```python
from build123d import *

# Parameters (mm, degrees)
F0_R     = 1.75
F1_DEPTH = 12
F2_R     = 1.75
F3_DEPTH = 15


with BuildPart() as f1:
    # F0 (on Top) → F1 (new body)
    with BuildSketch(Plane.XY):
        Polygon((160, 0), (0, 0), (0, -25), (42, -25), (42, -120), (110, -120), (110, -50), (160, -50), align=None)
        with Locations((49, -113)):
            Circle(F0_R, mode=Mode.SUBTRACT)
        with Locations((103, -113)):
            Circle(F0_R, mode=Mode.SUBTRACT)
        with Locations((49, -59)):
            Circle(F0_R, mode=Mode.SUBTRACT)
        with Locations((9, -12.5)):
            Circle(F0_R, mode=Mode.SUBTRACT)
        with Locations((103, -59)):
            Circle(F0_R, mode=Mode.SUBTRACT)
        with Locations((111, -12.5)):
            Circle(F0_R, mode=Mode.SUBTRACT)
        with Locations((141, -8)):
            Circle(F0_R, mode=Mode.SUBTRACT)
    extrude(amount=F1_DEPTH)

    # F2 (on face) → F3 (cut)
    with BuildSketch(Plane(origin=(0, 0, 0), x_dir=(-1, 0, 0), z_dir=(0, 1, 0))):
        with Locations((-156, 6)):
            Circle(F2_R)
        with Locations((-84, 6)):
            Circle(F2_R)
        with Locations((-13, 6)):
            Circle(F2_R)
    extrude(amount=-F3_DEPTH, mode=Mode.SUBTRACT)


solid = f1.part
```
Could you check a few things on this model? Use its own coordinates, in mm. A direction names the side the tool comes from. Give positions to 0.01 mm unless a question says otherwise; leave off trailing zeros. Order: outer loops, then holes, each group sorted by start corner. A loop starts at its lowest first (then second) coordinate and runs counter-clockwise, first axis right, second up.
Q1. For faces 1 (the flat face through (42, -72, 6)), 2 (the flat face through (135, -50, 6)), 3 (the cylindrical face through (82.331, -7.395, 6.526)), which set-ups out of +Z, -Z, +X, -X, +Y, -Y let a thin tool reach every point of the face, with its end or its side?
Q2. If I drill on line 1 along X through (y, z) = (-113, 3.5); line 2 along Y through (x, z) = (49, 8); line 3 along Y through (x, z) = (111, 4), over which ranges is the centre line in solid material (lowest first)?
Q3. Suppose I cut it at A-A, the plane x = 49. Write out the boundary of the cut face in (y, z), and give its area (3 significant figures).
Q4. Suppose I cut it at D-D, the plane x = 13. Write out the boundary of the cut face in (y, z), and give its area (4 significant figures).
Q5. Suppose I cut it at C-C, the plane y = -59. Write out the boundary of the cut face in (x, z), and give its area (3 significant figures).
Q6. Suppose I cut it at B-B, the plane y = -8. Write out the boundary of the cut face in (x, z), and give its area (3 significant figures).
Q7. I'm going to push flat-ended pins straight in: P1, Ø4, axis at y = -75, z = 3, coming from the -X side; P2, Ø4, axis at x = 156, z = 6, coming from the -Y side; P3, Ø5, axis at x = 28, z = 5, coming from the -Y side. Where does each tip first touch, or does it pass through?
Q8. We'd pull the mould along Z, two halves only. Please class faces 4 (the cylindrical face through (12.19, -7.4, 4.45)), 5 (the flat face through (110, -85, 6)), 6 (the flat face through (79, -46, 0)): +Z half, -Z half, draft (parallel to the pull), parting line (faces both ways), or undercut.
Solution:
1. face 1: +Z, -Z, -X, -Y
1. face 2: +Z, -Z, +X, -Y
1. face 3: +Y
2. line 1: x = 42 to 47.25, 50.75 to 101.25, 104.75 to 110
2. line 2: y = -120 to -114.75, -111.25 to -60.75, -57.25 to 0
2. line 3: y = -50 to -14.25, -10.75 to 0
3. outline: (-120, 0) - (-114.75, 0) - (-114.75, 12) - (-120, 12) - close; (-111.25, 0) - (-60.75, 0) - (-60.75, 12) - (-111.25, 12) - close; (-57.25, 0) - (0, 0) - (0, 12) - (-57.25, 12) - close
3. area: 1,360 mm2
4. outline: (-25, 0) - (0, 0) - (0, 4.25) - (-15, 4.25) - (-15, 7.75) - (0, 7.75) - (0, 12) - (-25, 12) - close
4. area: 247.5 mm2
5. outline: (42, 0) - (47.25, 0) - (47.25, 12) - (42, 12) - close; (50.75, 0) - (101.25, 0) - (101.25, 12) - (50.75, 12) - close; (104.75, 0) - (110, 0) - (110, 12) - (104.75, 12) - close
5. area: 732 mm2
6. outline: (0, 0) - (139.25, 0) - (139.25, 12) - (0, 12) - close; (142.75, 0) - (160, 0) - (160, 12) - (142.75, 12) - close; hole circle Ø3.5 at (13, 6); hole circle Ø3.5 at (84, 6); hole circle Ø3.5 at (156, 6)
6. area: 1,850 mm2
7. P1: stops at x = 42
7. P2: stops at y = -50
7. P3: stops at y = -25
8. face 4: undercut
8. face 5: draft
8. face 6: -Z half
